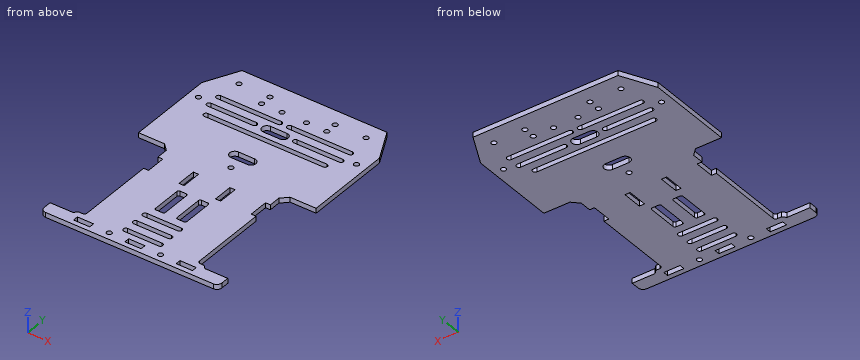
from build123d import *

# Parameters (mm, degrees)
ESBO_O1_R                = 1.55
ESBO_O1_W                = 3.2
ESBO_O1_H                = 12
ESBO_O1_W_2              = 10
ESBO_O1_H_2              = 3.2
RESSALTO_EXTRUS_O1_DEPTH = 3
ESBO_O2_R                = 1.55
CORTE_EXTRUS_O1_DEPTH    = 10
ESBO_O3_R                = 1.55
CORTE_EXTRUS_O2_DEPTH    = 190.512532567
CORTE_EXTRUS_O5_DEPTH    = 10


with BuildPart() as part:
    # Esboço1 → Ressalto-extrusão1 (new body)
    with BuildSketch(Plane.XY):
        with BuildLine():
            Line((0, 82), (16, 82))
            Line((16, 82), (20, 78))
            Line((20, 78), (20, 71))
            Line((20, 71), (23, 71))
            Line((23, 71), (23, 59))
            Line((23, 59), (20, 59))
            Line((20, 59), (20, 11.5))
            ThreePointArc((20, 11.5), (19.560660172, 10.439339828), (18.5, 10))
            Line((18.5, 10), (16, 10))
            Line((16, 10), (14, 8))
            Line((14, 8), (0, 8))
            Line((0, 8), (0, 3))
            ThreePointArc((0, 3), (0.878679656, 0.878679656), (3, 0))
            Line((3, 0), (106, 0))
            ThreePointArc((106, 0), (108.121320344, 0.878679656), (109, 3))
            Line((109, 3), (109, 8))
            Line((109, 8), (95, 8))
            Line((95, 8), (93, 10))
            Line((93, 10), (90.5, 10))
            ThreePointArc((90.5, 10), (89.439339828, 10.439339828), (89, 11.5))
            Line((89, 11.5), (89, 59))
            Line((89, 59), (86, 59))
            Line((86, 59), (86, 71))
            Line((86, 71), (89, 71))
            Line((89, 71), (89, 78))
            Line((89, 78), (93, 82))
            Line((93, 82), (109, 82))
            Line((109, 82), (109, 135))
            Line((109, 135), (99, 155))
            Line((99, 155), (10, 155))
            Line((10, 155), (0, 135))
            Line((0, 135), (0, 82))
        make_face()
        with Locations((47, 138)):
            Circle(ESBO_O1_R, mode=Mode.SUBTRACT)
        with Locations((62, 138)):
            Circle(ESBO_O1_R, mode=Mode.SUBTRACT)
        with Locations((74.5, 138)):
            Circle(ESBO_O1_R, mode=Mode.SUBTRACT)
        with Locations((34.5, 138)):
            Circle(ESBO_O1_R, mode=Mode.SUBTRACT)
        with Locations((74.5, 145)):
            Circle(ESBO_O1_R, mode=Mode.SUBTRACT)
        with Locations((93.5, 145)):
            Circle(ESBO_O1_R, mode=Mode.SUBTRACT)
        with Locations((15.5, 145)):
            Circle(ESBO_O1_R, mode=Mode.SUBTRACT)
        with Locations((34.5, 145)):
            Circle(ESBO_O1_R, mode=Mode.SUBTRACT)
        with BuildLine():
            Line((59.1, 54), (63.1, 54))
            ThreePointArc((63.1, 54), (63.807106781, 53.707106781), (64.1, 53))
            Line((64.1, 53), (64.1, 35))
            ThreePointArc((64.1, 35), (63.807106781, 34.292893219), (63.1, 34))
            Line((63.1, 34), (59.1, 34))
            ThreePointArc((59.1, 34), (58.392893219, 34.292893219), (58.1, 35))
            Line((58.1, 35), (58.1, 53))
            ThreePointArc((58.1, 53), (58.392893219, 53.707106781), (59.1, 54))
        make_face(mode=Mode.SUBTRACT)
        with Locations((43.3, 65)):
            Rectangle(ESBO_O1_W, ESBO_O1_H, mode=Mode.SUBTRACT)
        with Locations((65.7, 65)):
            Rectangle(ESBO_O1_W, ESBO_O1_H, mode=Mode.SUBTRACT)
        with BuildLine():
            Line((45.9, 54), (49.9, 54))
            ThreePointArc((49.9, 54), (50.607106781, 53.707106781), (50.9, 53))
            Line((50.9, 53), (50.9, 35))
            ThreePointArc((50.9, 35), (50.607106781, 34.292893219), (49.9, 34))
            Line((49.9, 34), (45.9, 34))
            ThreePointArc((45.9, 34), (45.192893219, 34.292893219), (44.9, 35))
            Line((44.9, 35), (44.9, 53))
            ThreePointArc((44.9, 53), (45.192893219, 53.707106781), (45.9, 54))
        make_face(mode=Mode.SUBTRACT)
        with Locations((86, 4.6)):
            Rectangle(ESBO_O1_W_2, ESBO_O1_H_2, mode=Mode.SUBTRACT)
        with Locations((54.5, 4.6)):
            Rectangle(ESBO_O1_W_2, ESBO_O1_H_2, mode=Mode.SUBTRACT)
        with Locations((23, 4.6)):
            Rectangle(ESBO_O1_W_2, ESBO_O1_H_2, mode=Mode.SUBTRACT)
    extrude(amount=RESSALTO_EXTRUS_O1_DEPTH)

    # Esboço2 → Corte-extrusão1 (cut)
    with BuildSketch(Plane(origin=(0, 0, 0), x_dir=(-1, 0, 0), z_dir=(0, 0, -1))):
        with Locations((-54.5, 85)):
            Circle(ESBO_O2_R)
        with Locations((-70.25, 4.6)):
            Circle(ESBO_O2_R)
        with Locations((-38.75, 4.6)):
            Circle(ESBO_O2_R)
    extrude(amount=-CORTE_EXTRUS_O1_DEPTH, mode=Mode.SUBTRACT)

    # Esboço3 → Corte-extrusão2 (cut, through all)
    with BuildSketch(Plane.XY.offset(3)):
        with Locations((6, 124)):
            Circle(ESBO_O3_R)
        with Locations((103, 124)):
            Circle(ESBO_O3_R)
    extrude(amount=-CORTE_EXTRUS_O2_DEPTH, mode=Mode.SUBTRACT)

    # Esboço5 → Corte-extrusão5 (cut)
    with BuildSketch(Plane(origin=(0, 0, 0), x_dir=(-1, 0, 0), z_dir=(0, 0, -1))):
        with BuildLine():
            Line((-95, 131.5), (-57.5, 131.5))
            ThreePointArc((-57.5, 131.5), (-56, 130), (-57.5, 128.5))
            Line((-57.5, 128.5), (-95, 128.5))
            ThreePointArc((-95, 128.5), (-96.5, 130), (-95, 131.5))
        make_face()
        with BuildLine():
            Line((-51.5, 131.5), (-14, 131.5))
            ThreePointArc((-14, 131.5), (-12.5, 130), (-14, 128.5))
            Line((-14, 128.5), (-51.5, 128.5))
            ThreePointArc((-51.5, 128.5), (-53, 130), (-51.5, 131.5))
        make_face()
        with BuildLine():
            Line((-59.5, 125), (-49.5, 125))
            ThreePointArc((-49.5, 125), (-46.5, 122), (-49.5, 119))
            Line((-49.5, 119), (-59.5, 119))
            ThreePointArc((-59.5, 119), (-62.5, 122), (-59.5, 125))
        make_face()
        with BuildLine():
            Line((-95, 123.5), (-67, 123.5))
            ThreePointArc((-67, 123.5), (-65.5, 122), (-67, 120.5))
            Line((-67, 120.5), (-95, 120.5))
            ThreePointArc((-95, 120.5), (-96.5, 122), (-95, 123.5))
        make_face()
        with BuildLine():
            Line((-42, 123.5), (-14, 123.5))
            ThreePointArc((-14, 123.5), (-12.5, 122), (-14, 120.5))
            Line((-14, 120.5), (-42, 120.5))
            ThreePointArc((-42, 120.5), (-43.5, 122), (-42, 123.5))
        make_face()
        with BuildLine():
            Line((-91, 115.5), (-18, 115.5))
            ThreePointArc((-18, 115.5), (-16.5, 114), (-18, 112.5))
            Line((-18, 112.5), (-91, 112.5))
            ThreePointArc((-91, 112.5), (-92.5, 114), (-91, 115.5))
        make_face()
        with BuildLine():
            Line((-59.5, 98), (-49.5, 98))
            ThreePointArc((-49.5, 98), (-46.5, 95), (-49.5, 92))
            Line((-49.5, 92), (-59.5, 92))
            ThreePointArc((-59.5, 92), (-62.5, 95), (-59.5, 98))
        make_face()
        with BuildLine():
            Line((-65.1, 13), (-43.9, 13))
            ThreePointArc((-43.9, 13), (-42.4, 11.5), (-43.9, 10))
            Line((-43.9, 10), (-65.1, 10))
            ThreePointArc((-65.1, 10), (-66.6, 11.5), (-65.1, 13))
        make_face()
        with BuildLine():
            Line((-65.1, 21), (-43.9, 21))
            ThreePointArc((-43.9, 21), (-42.4, 19.5), (-43.9, 18))
            Line((-43.9, 18), (-65.1, 18))
            ThreePointArc((-65.1, 18), (-66.6, 19.5), (-65.1, 21))
        make_face()
        with BuildLine():
            Line((-65.1, 29), (-43.9, 29))
            ThreePointArc((-43.9, 29), (-42.4, 27.5), (-43.9, 26))
            Line((-43.9, 26), (-65.1, 26))
            ThreePointArc((-65.1, 26), (-66.6, 27.5), (-65.1, 29))
        make_face()
    extrude(amount=-CORTE_EXTRUS_O5_DEPTH, mode=Mode.SUBTRACT)


solid = part.part
Geometry: final body of the model. Coordinates: model frame, mm. Give positions to 0.01 mm unless a question says otherwise; leave off trailing zeros. Loops run counter-clockwise (first coordinate to the right, second up) from the corner with the lowest first, then second, coordinate; pieces in that order, holes last. Notation, with made-up numbers: (3.5, 82.25) - (53.5, 82.25) arc R26 ccw to (53.5, 115.25) - close; hole circle Ø3 at (1.5, 52.25). An arc over 180 degrees is marked (long way). One line per question, with ' | ' between items. Start each with the question number.
(1) Section query A-A on x = 38.75. Return loops of the section in (y, z), then the cut area to 3 significant figures.
(2) Section query B-B on y = 96. Return loops of the section in (x, z).
(3) Section query C-C on z = 1.1. Count the separate pieces of the cut face and the enclosed holes in it, then the cut area to 3 significant figures.
(4) Contact query for flat-ended pins moving along their axis: pin 1 (0.9 mm diameter, centred on y = 34, z = 2, fed in from +X); pin 2 (0.9 mm diameter, centred on y = 45.5, z = 2, fed in from -X); pin 3 (0.9 mm diameter, centred on y = 62, z = 1, fed in from -X). Output: stop coordinate, or through.
(5) Ray query, line 1 (Y direction, x = 39, z = 0.5); line 2 (X direction, y = 66, z = 1.4); line 3 (Y direction, x = 74.5, z = 2.25). Return the intervals inside material, ascending. Write a range as from..to.
The answers:
1) outline: (0, 0) - (3.05, 0) - (3.05, 3) - (0, 3) - close; (6.15, 0) - (112.5, 0) - (112.5, 3) - (6.15, 3) - close; (115.5, 0) - (120.5, 0) - (120.5, 3) - (115.5, 3) - close; (123.5, 0) - (128.5, 0) - (128.5, 3) - (123.5, 3) - close; (131.5, 0) - (155, 0) - (155, 3) - (131.5, 3) - close | area: 429 mm2
2) outline: (0, 0) - (46.67, 0) - (46.67, 3) - (0, 3) - close; (62.33, 0) - (109, 0) - (109, 3) - (62.33, 3) - close
3) separate pieces: 1 | enclosed holes: 30 | area: 12,200 mm2
4) pin 1: x = 89 | pin 2: x = 20 | pin 3: x = 23
5) line 1: 0..3.07, 6.13..112.5, 115.5..120.5, 123.5..128.5, 131.5..155 | line 2: 23..41.7, 44.9..64.1, 67.3..86 | line 3: 0..112.5, 115.5..120.5, 123.5..128.5, 131.5..136.45, 139.55..143.45, 146.55..155
